Here's how the part is built. I have some questions about the finished solid (model axes, mm). Face numbers are marked on the shaded views. A direction names the side the tool comes from. Coordinates: 2 decimals unless noted, no trailing zeros. Loops run counter-clockwise (first coordinate to the right, second up) from the corner with the lowest first, then second, coordinate; pieces in that order, holes last. Notation, with made-up numbers: (-26, 44) - (-7, 44) arc R22 cw to (-7, 65) - close; hole circle Ø6 at (50, 17). An arc over 180 degrees is marked (long way). Use a Markdown table: item, result.
```python
from build123d import *

# Parameters (mm, degrees)
SKETCH1_W           = 44.85
SKETCH1_H           = 44.85
SKETCH1_W_2         = 38.5
SKETCH1_H_2         = 38.5
BOSS_EXTRUDE1_DEPTH = 19.25
SKETCH2_W           = 44.85
SKETCH2_H           = 44.85
BOSS_EXTRUDE2_DEPTH = 3.175
SKETCH3_W           = 44.85
SKETCH3_H           = 44.85
BOSS_EXTRUDE3_DEPTH = 3.175
SKETCH5_R           = 12.7
CUT_EXTRUDE1_DEPTH  = 3.175
CUT_EXTRUDE2_START  = 22.425
SKETCH6_R           = 10
CUT_EXTRUDE2_DEPTH  = 41.675
SKETCH7_R           = 12.7
CUT_EXTRUDE3_DEPTH  = 55.929807482
SKETCH8_W           = 44.85
SKETCH8_H           = 44.85
SKETCH8_R           = 2.2225
BOSS_EXTRUDE4_DEPTH = 6.35
SKETCH9_R           = 3.4925
CUT_EXTRUDE4_DEPTH  = 6.35
CUT_EXTRUDE5_REACH  = 62.226
SKETCH10_W          = 38.5
SKETCH10_H          = 38.5
SKETCH11_R          = 12.1285
BOSS_EXTRUDE5_DEPTH = 25.4
CUT_EXTRUDE6_START  = 47.825
CUT_EXTRUDE6_DEPTH  = 2.54


with BuildPart() as part:
    # Sketch1 → Boss-Extrude1 (new, symmetric)
    with BuildSketch(Plane(origin=(0, 0, 0), x_dir=(1, 0, 0), z_dir=(0, 1, 0))):
        Rectangle(SKETCH1_W, SKETCH1_H)
        Rectangle(SKETCH1_W_2, SKETCH1_H_2, mode=Mode.SUBTRACT)
    extrude(amount=BOSS_EXTRUDE1_DEPTH, both=True)

    # Sketch2 → Boss-Extrude2 (add)
    with BuildSketch(Plane(origin=(0, 19.25, 0), x_dir=(1, 0, 0), z_dir=(0, 1, 0))):
        Rectangle(SKETCH2_W, SKETCH2_H)
    extrude(amount=BOSS_EXTRUDE2_DEPTH)

    # Sketch3 → Boss-Extrude3 (add)
    with BuildSketch(Plane.XZ.offset(19.25)):
        Rectangle(SKETCH3_W, SKETCH3_H)
    extrude(amount=BOSS_EXTRUDE3_DEPTH)

    # Sketch5 → Cut-Extrude1 (cut)
    with BuildSketch(Plane(origin=(0, -22.425, -22.425), x_dir=(1, 0, 0), z_dir=(0, 1, 0))):
        with Locations(Location((0, -22.425, 0), (0, 0, 90))):
            Circle(SKETCH5_R)
    extrude(amount=CUT_EXTRUDE1_DEPTH, mode=Mode.SUBTRACT)

    # Sketch6 → Cut-Extrude2 (cut)
    with BuildSketch(Plane(origin=(0, 0, 0), x_dir=(1, 0, 0), z_dir=(0, 1, 0)).offset(CUT_EXTRUDE2_START)):
        with Locations(Location((0, 0, 0), (0, 0, 270))):
            Circle(SKETCH6_R)
    extrude(amount=-CUT_EXTRUDE2_DEPTH, mode=Mode.SUBTRACT)

    # Sketch7 → Cut-Extrude3 (cut, through all)
    with BuildSketch(Plane.ZY.offset(22.425)):
        Circle(SKETCH7_R)
    extrude(amount=-CUT_EXTRUDE3_DEPTH, mode=Mode.SUBTRACT)

    # Sketch8 → Boss-Extrude4 (add)
    with BuildSketch(Plane(origin=(0, 0, -22.425), x_dir=(-1, 0, 0), z_dir=(0, 0, -1))):
        Rectangle(SKETCH8_W, SKETCH8_H)
        with Locations((-12.7, 12.7)):
            Circle(SKETCH8_R, mode=Mode.SUBTRACT)
        with Locations((0, 12.7)):
            Circle(SKETCH8_R, mode=Mode.SUBTRACT)
        with Locations((12.7, 12.7)):
            Circle(SKETCH8_R, mode=Mode.SUBTRACT)
        Circle(SKETCH8_R, mode=Mode.SUBTRACT)
        with Locations((12.7, 0)):
            Circle(SKETCH8_R, mode=Mode.SUBTRACT)
        with Locations((0, -12.7)):
            Circle(SKETCH8_R, mode=Mode.SUBTRACT)
        with Locations((12.7, -12.7)):
            Circle(SKETCH8_R, mode=Mode.SUBTRACT)
        with Locations((-12.7, 0)):
            Circle(SKETCH8_R, mode=Mode.SUBTRACT)
        with Locations((-12.7, -12.7)):
            Circle(SKETCH8_R, mode=Mode.SUBTRACT)
    extrude(amount=BOSS_EXTRUDE4_DEPTH)

    # Sketch9 → Cut-Extrude4 (cut)
    with BuildSketch(Plane.XY.offset(-19.25)):
        with Locations((12.7, 12.7)):
            Circle(SKETCH9_R)
        with Locations((0, 12.7)):
            Circle(SKETCH9_R)
        with Locations((-12.7, 12.7)):
            Circle(SKETCH9_R)
        Circle(SKETCH9_R)
        with Locations((-12.7, 0)):
            Circle(SKETCH9_R)
        with Locations((0, -12.7)):
            Circle(SKETCH9_R)
        with Locations((-12.7, -12.7)):
            Circle(SKETCH9_R)
        with Locations((12.7, 0)):
            Circle(SKETCH9_R)
        with Locations((12.7, -12.7)):
            Circle(SKETCH9_R)
    extrude(amount=-CUT_EXTRUDE4_DEPTH, mode=Mode.SUBTRACT)

    # Sketch10 → Cut-Extrude5 (cut, up to next)
    with BuildSketch(Plane.XY.offset(22.425), mode=Mode.PRIVATE) as cut_extrude5_sk1:
        Rectangle(SKETCH10_W, SKETCH10_H)
    cut_extrude5_tool1 = extrude(cut_extrude5_sk1.sketch, amount=-CUT_EXTRUDE5_REACH, mode=Mode.PRIVATE) & part.part
    add(cut_extrude5_tool1.solids().sort_by_distance((0, 0, 22.425))[0], mode=Mode.SUBTRACT)

    # Sketch11 → Boss-Extrude5 (add)
    with BuildSketch(Plane(origin=(0, 22.425, 0), x_dir=(1, 0, 0), z_dir=(0, 1, 0))):
        with BuildLine():
            Line((-15.3035, 0), (-15.3035, 28.775))
            Line((-15.3035, 28.775), (15.3035, 28.775))
            Line((15.3035, 28.775), (15.3035, 0))
            ThreePointArc((15.3035, 0), (0, -15.3035), (-15.3035, 0))
        make_face()
        with Locations(Location((0, 0, 0), (0, 0, 270))):
            Circle(SKETCH11_R, mode=Mode.SUBTRACT)
    extrude(amount=BOSS_EXTRUDE5_DEPTH)

    # Sketch12 → Cut-Extrude6 (cut)
    with BuildSketch(Plane(origin=(0, 0, 0), x_dir=(1, 0, 0), z_dir=(0, 1, 0)).offset(CUT_EXTRUDE6_START)):
        Polygon((-7.032749725, 23.499615385), (-5.176595879, 23.499615385), (-3.255313828, 19.117708333), (-1.334031776, 23.499615385), (0.52212207, 23.499615385), (-2.730217674, 16.075), (-3.780409982, 16.075), align=None)
        with BuildLine():
            Line((3.06212207, 22.848333333), (1.238532326, 22.848333333))
            add(Edge.make_bspline(
                [(1.238532326, 22.848333333), (1.246408131, 22.98627825), (1.26179698, 23.255814335), (1.323009931, 23.647324128), (1.405033186, 24.017257831), (1.514504108, 24.364321375), (1.652061484, 24.688388647), (1.814165609, 24.990564412), (2.004957875, 25.269257707), (2.220377594, 25.523124515), (2.456767534, 25.750870772), (2.709220005, 25.95280491), (2.98159661, 26.119435879), (3.268920804, 26.25655774), (3.571143663, 26.366111735), (3.891124689, 26.439357446), (4.226093313, 26.488960159), (4.455406461, 26.493300596), (4.572282326, 26.495512821)],
                knots=[0, 0, 0, 0, 1.199038563, 2.342849363, 3.436047546, 4.486744587, 5.497670872, 6.488682221, 7.459191391, 8.424610317, 9.374430501, 10.305433194, 11.225809216, 12.140057399, 13.06607119, 14.010487599, 14.985989317, 16, 16, 16, 16], degree=3))
            add(Edge.make_bspline(
                [(4.572282326, 26.495512821), (4.715745792, 26.491036382), (4.995820098, 26.482297326), (5.402790279, 26.407750272), (5.782855932, 26.283058805), (6.135740783, 26.108831941), (6.458440664, 25.887494974), (6.75090206, 25.623586865), (7.004280474, 25.311570683), (7.220182398, 24.964428914), (7.399571093, 24.596854636), (7.525279218, 24.216767589), (7.607905816, 23.834253744), (7.616718454, 23.576688282), (7.621096429, 23.448733974)],
                knots=[0, 0, 0, 0, 1.075374347, 2.099382735, 3.09057751, 4.06680945, 5.040638231, 6.016817125, 7.011024321, 8.044445721, 9.0776792, 10.070479129, 11.0414456, 12, 12, 12, 12], degree=3))
            add(Edge.make_bspline(
                [(7.621096429, 23.448733974), (7.619391877, 23.371338166), (7.615961034, 23.215559521), (7.592105933, 22.979828197), (7.556318567, 22.739708284), (7.50235994, 22.495405661), (7.435069108, 22.246851846), (7.353435604, 21.993303005), (7.255565857, 21.736196664), (7.143093114, 21.472639138), (7.008912847, 21.201774756), (6.852678577, 20.919543158), (6.670243493, 20.626194704), (6.463811181, 20.320073055), (6.232379047, 20.00166101), (5.974817317, 19.671917726), (5.694092498, 19.329681294), (5.494854196, 19.100915445), (5.392490659, 18.98338141)],
                knots=[0, 0, 0, 0, 0.728284026, 1.46585585, 2.227944881, 3.01186502, 3.81876927, 4.650621989, 5.517437689, 6.406905708, 7.346299482, 8.360816762, 9.441613733, 10.596154504, 11.834900912, 13.145207542, 14.533280747, 16, 16, 16, 16], degree=3))
            Line((5.392490659, 18.98338141), (4.33212207, 17.768333333))
            Line((4.33212207, 17.768333333), (7.751352839, 17.768333333))
            Line((7.751352839, 17.768333333), (7.751352839, 16.075))
            Line((7.751352839, 16.075), (0.978019506, 16.075))
            Line((0.978019506, 16.075), (0.978019506, 16.99900641))
            Line((0.978019506, 16.99900641), (3.98612848, 20.200464744))
            add(Edge.make_bspline(
                [(3.98612848, 20.200464744), (4.073220965, 20.293852277), (4.241893281, 20.474716236), (4.481896603, 20.7403342), (4.69907841, 20.992399308), (4.888935258, 21.233595544), (5.061430592, 21.456099485), (5.208872858, 21.666617676), (5.332611037, 21.863246958), (5.46694638, 22.10034753), (5.594520797, 22.383132155), (5.711578046, 22.708911637), (5.782932539, 23.020281793), (5.792781716, 23.22317728), (5.797506685, 23.320512821)],
                knots=[0, 0, 0, 0, 1.246127091, 2.413378631, 3.493388633, 4.492180848, 5.408488754, 6.240484944, 6.999099869, 7.674939598, 8.898438119, 10.020720584, 11.050475521, 12, 12, 12, 12], degree=3))
            add(Edge.make_bspline(
                [(5.797506685, 23.320512821), (5.79397394, 23.414677447), (5.787128679, 23.597136506), (5.711904814, 23.856683548), (5.595365392, 24.091676899), (5.431144887, 24.295094693), (5.232222423, 24.462256582), (5.002348831, 24.5865869), (4.743398255, 24.658324923), (4.561868968, 24.667303961), (4.468484249, 24.671923077)],
                knots=[0, 0, 0, 0, 1.062038974, 2.057870785, 3.028805853, 4.01125022, 4.991535629, 5.949134679, 6.94496649, 8, 8, 8, 8], degree=3))
            add(Edge.make_bspline(
                [(4.468484249, 24.671923077), (4.420240514, 24.67021672), (4.325264974, 24.666857482), (4.185658353, 24.644495946), (4.052812623, 24.605086073), (3.925249138, 24.552282391), (3.804329288, 24.48229073), (3.690358071, 24.396014857), (3.582134658, 24.295647238), (3.480155402, 24.181501708), (3.387340967, 24.054115264), (3.304903526, 23.91465132), (3.236741485, 23.763196445), (3.176729147, 23.601750075), (3.13044476, 23.428578144), (3.096743985, 23.244717066), (3.071123536, 23.050465961), (3.065177143, 22.916936592), (3.06212207, 22.848333333)],
                knots=[0, 0, 0, 0, 0.903469896, 1.778625579, 2.63899355, 3.493148037, 4.358286772, 5.247621495, 6.164656832, 7.118446693, 8.109501108, 9.111810964, 10.146451449, 11.215617525, 12.33435995, 13.498009769, 14.714554818, 16, 16, 16, 16], degree=3))
        make_face()
    extrude(amount=-CUT_EXTRUDE6_DEPTH, mode=Mode.SUBTRACT)


solid = part.part
```
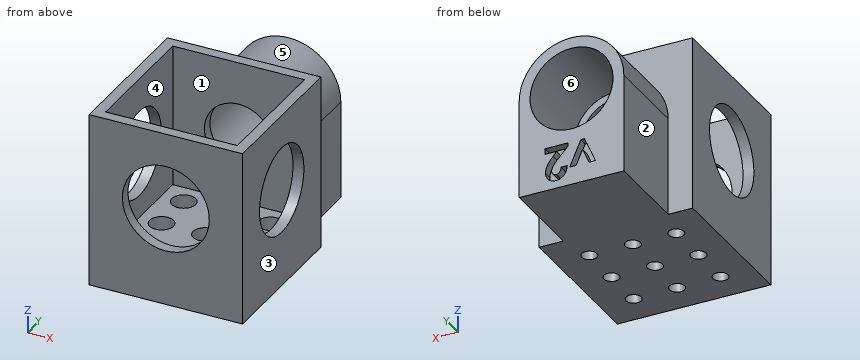
Q1. Which directions (+Z, -Z, +X, -X, +Y, -Y) give clear straight access to the entire face, cutting with the end or side of a thin tool? Please do the marked faces 4, 5 and 6.
Check values:
| item | result |
|---|---|
| face 4 | +Z |
| face 5 | +Z, +Y |
| face 6 | +Y |
Q2. Will these pins go through, and if not, where does the flat tip stop? P1, Ø3.5, axis at x = 6, z = -21.5, coming from the +Y side (3 decimals); P2, Ø12, axis at y = 39, z = 11.5, coming from the +X side; P3, Ø3.5, axis at x = 13.5, y = 1.5, coming from the +Z side; P4, Ø5.5, axis at x = 1, y = -14, coming from the +Z side.
Check values:
| item | result |
|---|---|
| P1 | y = 47.825 |
| P2 | x = 14.28 |
| P3 | z = -25.6 |
| P4 | z = -19.25 |
Q3. If we mould it in two halves opening along X, with no side actions, what happens to the marked faces 1, 2 and 3? For each: pulls with the +X half, pulls with the -X half, needs draft (parallel to the pull), parting line crosses it, or undercut.
Check values:
| item | result |
|---|---|
| face 1 | undercut |
| face 2 | pulls with the -X half |
| face 3 | pulls with the +X half |
Q4. Please list where these lines run through material, in increasing order: L1, parallel to Y at x = -12.7, z = -24 (1 decimal); L2, parallel to Y at x = 6, z = -12 (3 decimals); L3, parallel to Y at x = -16.5, z = 13 (3 decimals). Write a range as from..to.
Check values:
| item | result |
|---|---|
| L1 | -22.4..-16.2, -9.2..-3.5, 3.5..9.2, 16.2..47.8 |
| L2 | -22.425..-19.25, 19.25..47.825 |
| L3 | -22.425..-19.25, 19.25..22.425 |
Q5. I want a section at B-B, the plane x = -17. Write out the boundary of the cut face in (y, z) (3 decimals), then the cut area to 3 significant figures.
Check values:
| item | result |
|---|---|
| outline | (-22.425, -28.775) - (22.425, -28.775) - (22.425, 22.425) - (19.25, 22.425) - (19.25, -19.25) - (-19.25, -19.25) - (-19.25, 22.425) - (-22.425, 22.425) - close |
| area | 692 mm^2 |
Q6. I want a section at A-A, the plane z = -8.5. Give the number of separate pieces and of enclosed holes in the cut face, then the cut area to 3 significant figures.
Check values:
| item | result |
|---|---|
| separate pieces | 4 |
| enclosed holes | 0 |
| area | 654 mm^2 |
